Work out the finished part from the listing and answer in its coordinate system (mm). Face numbers are marked on the shaded views. A direction names the side the tool comes from. Give positions to 0.01 mm unless a question says otherwise; leave off trailing zeros. Loops run counter-clockwise (first coordinate to the right, second up) from the corner with the lowest first, then second, coordinate; pieces in that order, holes last. Notation, with made-up numbers: M -12,22 L 43,22 A14 cw 43,45 Z; hole C 70.5,70 d5. An arc over 180 degrees is marked long. Use a Markdown table: item, result.
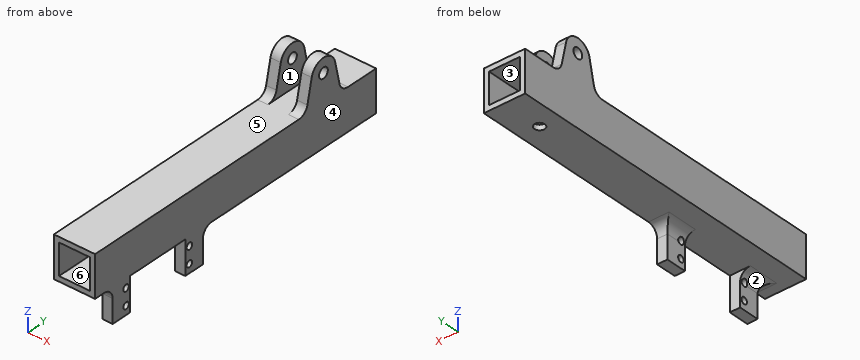
Autodesk Inventor part; units mm, degrees
ref_plane "Work Plane1" through (12.7, 0, 0) normal (1, 0, 0) x (0, 0, -1)
ref_plane "YZ Plane" through (0, 0, 0) normal (1, 0, 0) x (0, 1, 0)
ref_plane "XZ Plane" through (0, 0, 0) normal (0, 1, 0) x (-1, 0, 0)
sketch "Sketch2" plane through (0, 0, 0) normal (0, 1, 0) x (-1, 0, 0)
  line L0 (0, 0) -> (-25.4, 0)
  line L1 (-25.4, 0) -> (-25.4, -25.4)
  line L2 (-25.4, -25.4) -> (0, -25.4)
  line L3 (0, -25.4) -> (0, 0)
  line L4 (-3.175, -22.225) -> (-22.225, -22.225)
  line L5 (-22.225, -22.225) -> (-22.225, -3.175)
  line L6 (-22.225, -3.175) -> (-3.175, -3.175)
  line L7 (-3.175, -3.175) -> (-3.175, -22.225)
  dimension "d4" = 3.175
  dimension "d5" = 3.175
  dimension "d6" = 19.05
  dimension "d7" = 19.05
  dimension "d8" = 3.175
  dimension "d9" = 3.175
extrude "Extrusion1" add sketch "Sketch2" along normal blind 203.2
sketch "Sketch3" plane through (25.4, 0, 0) normal (1, 0, 0) x (0, 0, -1)
  line L0 (0, 0) -> (25.4, 0)
  line L1 (25.4, 0) -> (25.4, 203.2)
  line L2 (25.4, 12.7) -> (46.2, 12.7)
  line L3 (46.2, 12.7) -> (46.2, 25.4)
  line L4 (46.2, 25.4) -> (25.4, 25.4)
  line L5 (25.4, 25.4) -> (25.4, 12.7)
  line L6 (25.4, 65.2112) -> (46.2, 65.2112)
  line L7 (46.2, 65.2112) -> (46.2, 77.9112)
  line L8 (46.2, 77.9112) -> (25.4, 77.9112)
  line L9 (25.4, 77.9112) -> (25.4, 65.2112)
  dimension "d12" = 39.8112
  dimension "d13" = 20.8
  dimension "d14" = 12.7
  dimension "d15" = 12.7
extrude "Extrusion2" add sketch "Sketch3" against normal blind 6.35
fillet "Fillet1" radius 6.35 4 edges at (22.225, 77.9112, -25.4) (22.225, 12.7, -25.4) (19.05, 19.05, -25.4) (19.05, 71.5612, -25.4)
sketch "Sketch4" plane through (25.4, 0, 0) normal (1, 0, 0) x (0, 0, -1)
  circle A0 centre (30.8, 68.2) radius 2
  circle A1 centre (40.8, 68.2) radius 2
  circle A2 centre (30.8, 22.4) radius 2
  circle A3 centre (40.8, 22.4) radius 2
  line L0 (46.2, 25.4) -> (25.4, 25.4)
  line L1 (25.4, 65.2112) -> (46.2, 65.2112)
  line L2 (46.2, 77.9112) -> (31.75, 77.9112)
  line L3 (25.4, 84.2612) -> (25.4, 203.2)
  line L4 (35.8, 65.2112) -> (35.8, 77.9112)
  dimension "d19" = 4
  dimension "d23" = 3
  dimension "d25" = 45.8
  dimension "d26" = 5
  dimension "d28" = 10
extrude "Extrusion3" cut sketch "Sketch4" against normal through all
sketch "Sketch5" plane through (25.4, 0, 0) normal (1, 0, 0) x (0, 0, -1)
  line L0 (0, 33.4612) -> (0, 203.2)
  line L1 (0, 177.8) -> (-19.05, 173.5767)
  line L2 (0, 152.4) -> (-19.05, 156.6233)
  arc A0 (-19.05, 173.5767) -> (-19.05, 156.6233) centre (-17.1708, 165.1) ccw
  circle A1 centre (-17.1708, 165.1) radius 3.175
  point P0 (0, -50.8)
  dimension "d29" = 25
  dimension "PivotWidth" = 25.4
  dimension "PivotHeight" = 19.05
  dimension "PivotAngle" = 102.5
  dimension "d33" = 203.2
  dimension "PivotScrewDiameter" = 6.35
extrude "Extrusion4" add sketch "Sketch5" against normal blind 6.35
ref_plane "Work Plane1" through (12.7, 0, 0) normal (1, 0, 0) x (0, 0, -1)
mirror "Mirror1" about plane through (12.7, 0, 0) normal (1, 0, 0) of "Extrusion4"
sketch "Sketch6" plane through (25.4, 177.8, 0) normal (0, 0.9763, 0.2164) x (1, 0, 0)
  line L0 (-19.05, 0) -> (-19.05, -19.5125)
  line L1 (-25.4, 0) -> (-25.4, -19.5125)
  line L2 (-25.4, 0) -> (-25.4, -19.5125)
  line L3 (-25.4, -19.5125) -> (-19.05, -19.5125)
  line L4 (-6.35, 0) -> (-6.35, -19.5125)
  point P0 (0, 6.35)
  point P1 (0, 0)
  point P2 (-25.4, -38.483)
  point P3 (0, 19.05)
  point P4 (6.35, -24.7979)
  point P5 (0, -24.7979)
  dimension "PivotOpeningWidth" = 12.7
fillet "Fillet3" radius 6.35 4 edges at (22.225, 177.8, 0) (3.175, 177.8, 0) (3.175, 152.4, 0) (22.225, 152.4, 0)
sketch "Sketch7" plane through (25.4, 0, -25.4) normal (0, 0, -1) x (-1, 0, 0)
  line L0 (25.4, 203.2) -> (0, 203.2)
  line L1 (12.7, 6.35) -> (12.7, 25.4)
  circle A0 centre (12.7, 177.8) radius 3.175
  line L2 (12.7, 203.2) -> (12.7, 165.4188)
  dimension "d40" = 6.35
  dimension "d41" = 25.4
extrude "Extrusion5" cut sketch "Sketch7" against normal blind 12.7
equation "\"d4\" = MastSupportWallThickness"
equation "\"d5\" = MastSupportWallThickness"
equation "\"d6\" = MastWidth"
equation "\"d7\" = MastWidth"
equation "\"d8\" = MastSupportWallThickness"
equation "\"d9\" = MastSupportWallThickness"
equation "\"d12\" = ServoLength + ServoTolerance"
equation "\"d13\" = ServoWidth + ServoTolerance"
equation "\"d23\" = ServoScrewOffsetFromSide - 0.5 * ServoTolerance"
equation "\"d25\" = ServoScrewSpacingLength"
equation "\"d26\" = 0.5 * ServerScrewSpacing"
equation "\"d28\" = ServerScrewSpacing"
equation "\"MastSupportWallThickness\" = 3.175"
equation "\"ServoLength\" = 38.8112"
equation "\"ServoWidth\" = 19.8"
equation "\"ServerScrewSpacing\" = 10"
equation "\"ServoScrewOffsetFromSide\" = 3.5"
equation "\"ServoScrewSpacingLength\" = 45.8"
equation "\"ServoTolerance\" = 1"
properties part number "TableMount-Base" material "ABS Plastic"
(1) The mould has two halves that part along Z. Classify the marked faces 4, 5 and 6: released by +Z, released by -Z, zero draft, split by the parting line, or undercut.
Entries:
| item | result |
|---|---|
| face 4 | zero draft |
| face 5 | released by +Z |
| face 6 | undercut |
(2) Which of the six approach directions +Z, -Z, +X, -X, +Y, -Y give full straight-line access (tool end or side, diameter ignored) to the marked faces 1, 2 and 3?
Entries:
| item | result |
|---|---|
| face 1 | +Z, +Y, -Y |
| face 2 | -Z, -X, +Y, -Y |
| face 3 | +Y, -Y |
(3) A cutting plane is placed at C-C (y = 105.5). Write down the section's boundary in (x, z) (3 decimals), and give its area (3 significant figures).
Entries:
| item | result |
|---|---|
| outline | M 0,-25.4 L 25.4,-25.4 L 25.4,0 L 0,0 Z; hole M 3.175,-22.225 L 22.225,-22.225 L 22.225,-3.175 L 3.175,-3.175 Z |
| area | 282 mm² |
(4) A cutting plane is placed at B-B (z = -40.8). Write down the section's boundary in (x, y).
Entries:
| item | result |
|---|---|
| outline | M 19.05,12.7 L 25.4,12.7 L 25.4,20.4 L 19.05,20.4 Z; M 19.05,24.4 L 25.4,24.4 L 25.4,25.4 L 19.05,25.4 Z; M 19.05,65.21 L 25.4,65.21 L 25.4,66.2 L 19.05,66.2 Z; M 19.05,70.2 L 25.4,70.2 L 25.4,77.91 L 19.05,77.91 Z |
(5) Consider probe 1 along Y at (x, z) = (19.75, -40.5); probe 2 along Z at (x, y) = (4, 165.1) (3 decimals); probe 3 along Y at (x, z) = (21, -36). Determine where each line is inside the solid, lowest interval first. Write a range as [from, to].
Entries:
| item | result |
|---|---|
| probe 1 | y = [12.7, 20.42], [24.38, 25.4], [65.21, 66.22], [70.18, 77.91] |
| probe 2 | z = [-25.4, -22.225], [-3.175, 13.996], [20.346, 25.853] |
| probe 3 | y = [12.7, 25.4], [65.21, 77.91] |
(6) A cutting plane is placed at D-D (z = 22.5). Write down the section's boundary in (x, y), and give its area (3 significant figures).
Entries:
| item | result |
|---|---|
| outline | M 0,158.25 L 6.35,158.25 L 6.35,171.95 L 0,171.95 Z; M 19.05,158.25 L 25.4,158.25 L 25.4,171.95 L 19.05,171.95 Z |
| area | 174 mm² |
(7) A cutting plane is placed at A-A (y = 68.2). Write down the section's boundary in (x, z) (3 decimals).
Entries:
| item | result |
|---|---|
| outline | M 0,-25.4 L 12.7,-25.4 A6.35 cw 18.323,-28.8 L 25.4,-28.8 L 25.4,0 L 0,0 Z; M 19.05,-46.2 L 25.4,-46.2 L 25.4,-42.8 L 19.05,-42.8 Z; M 19.05,-38.8 L 25.4,-38.8 L 25.4,-32.8 L 19.05,-32.8 Z; hole M 3.175,-22.225 L 22.225,-22.225 L 22.225,-3.175 L 3.175,-3.175 Z |
(8) Given P1, Ø1.9, axis at x = 21.5, z = -37.5, coming from the -Y side; P2, Ø6.5, axis at y = 69, z = -41.5, coming from the -X side; P3, Ø5.5, axis at x = 13.5, y = 88, coming from the +Z side, each flat-ended and moving along its own axis, determine where each tip first touches the part or whether it passes through.
Entries:
| item | result |
|---|---|
| P1 | stops at y = 12.7 |
| P2 | stops at x = 19.05 |
| P3 | stops at z = 0 |
